Geometry: final body of the model. Coordinates: model frame, mm. Face numbers are marked on the shaded views. Round coordinates to 2 decimals unless told otherwise and drop trailing zeros. Loops run counter-clockwise (first coordinate to the right, second up) from the corner with the lowest first, then second, coordinate; pieces in that order, holes last. Notation, with made-up numbers: (29, -7.75) -> (62, -7.75) arc R9 cw to (62, 4.25) -> close; hole circle Ø5 at (-9.75, 3). An arc over 180 degrees is marked (long way). Answer in a Markdown table with one row per item.
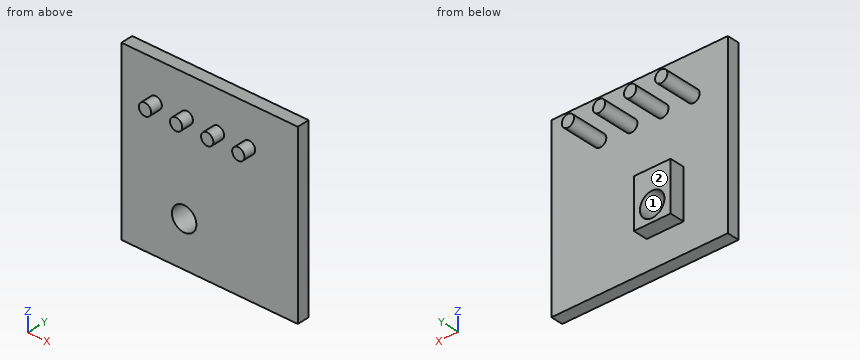
Autodesk Inventor part; units mm, degrees
ref_plane "YZ Plane" through (0, 0, 0) normal (1, 0, 0) x (0, 1, 0)
ref_plane "XZ Plane" through (0, 0, 0) normal (0, 1, 0) x (-1, 0, 0)
ref_plane "XY Plane" through (0, 0, 0) normal (0, 0, 1) x (1, 0, 0)
sketch "Skizze1" plane through (0, 0, 0) normal (0, 1, 0) x (-1, 0, 0)
  line L0 (0, 0) -> (14.4, 0)
  line L1 (14.4, 0) -> (14.4, -14.4)
  line L2 (14.4, -14.4) -> (0, -14.4)
  line L3 (0, -14.4) -> (0, 0)
  dimension "d0" = 14.4
  dimension "d1" = 14.4
extrude "Extrusion1" add sketch "Skizze1" along normal blind 1
sketch "Skizze2" plane through (0, 1, 0) normal (0, 1, 0) x (1, 0, 0)
  line L0 (0, 14.4) -> (-14.4, 14.4)
  line L1 (0, 0) -> (0, 14.4)
  point P0 (-9.28, 10.68)
  dimension "d4" = 3.72
  dimension "d5" = 9.28
hole "Bohrung1" at (-9.28, 1, -10.68) direction (0, -1, 0) diameter 2 end up to surface
sketch "Skizze3" plane through (0, 1, 0) normal (0, 1, 0) x (1, 0, 0)
  circle A0 centre (-9.28, 10.68) radius 1
  line L0 (-14.4, 0) -> (0, 0)
  line L1 (0, 0) -> (0, 14.4)
  line L2 (0, 14.4) -> (-14.4, 14.4)
  line L3 (-14.4, 14.4) -> (-14.4, 0)
  line L4 (-10.78, 8) -> (-7.78, 8)
  line L5 (-7.78, 8) -> (-7.78, 12)
  line L6 (-7.78, 12) -> (-10.78, 12)
  line L7 (-10.78, 12) -> (-10.78, 8)
  dimension "d13" = 4
  dimension "d14" = 3
  dimension "d15" = 1.5
  dimension "d16" = 1.32
extrude "Extrusion2" add sketch "Skizze3" along normal blind 1.2 contours L7 L6 L5 L4
sketch "Skizze4" plane through (0, 1, 0) normal (0, 1, 0) x (1, 0, 0)
  line L0 (-14.4, 14.4) -> (-14.4, 0) construction
  line L1 (-14.4, 3.2) -> (0, 3.2) construction
  line L2 (0, 0) -> (0, 14.4) construction
  line L3 (-14.4, 0) -> (0, 0)
  circle A0 centre (-11.6, 3.2) radius 0.5
  circle A1 centre (-9.06, 3.2) radius 0.5
  circle A2 centre (-6.52, 3.2) radius 0.5
  circle A3 centre (-3.98, 3.2) radius 0.5
  dimension "d19" = 3.2
  dimension "d20" = 2.8
  dimension "d21" = 2.54
  dimension "d22" = 2.54
  dimension "d23" = 2.54
  dimension "d24" = 1
  dimension "d25" = 1
  dimension "d26" = 1
  dimension "d27" = 1
extrude "Extrusion3" add sketch "Skizze4" along normal blind 3 and the other way blind 2
properties part number "Mic_breakout" material "ABS-Kunststoff"
Item 1: Section query D-D, the plane y = 3.4. Output: boundary loops of the cut face in (x, z), and give its area (3 significant figures).
Ans:
| item | result |
|---|---|
| outline | circle Ø1 at (-11.6, -3.2); circle Ø1 at (-9.06, -3.2); circle Ø1 at (-6.52, -3.2); circle Ø1 at (-3.98, -3.2) |
| area | 3.14 mm2 |
Item 2: Ray query, L1, parallel to X at y = 0.9, z = -10.68; L2, parallel to Z at x = -9.28, y = 0.8; L3, parallel to X at y = 3.3, z = -3.5. Return the intervals inside material, ascending.
Ans:
| item | result |
|---|---|
| L1 | -14.4 to -10.28, -8.28 to 0 |
| L2 | -14.4 to -11.68, -9.68 to 0 |
| L3 | -12 to -11.2, -9.46 to -8.66, -6.92 to -6.12, -4.38 to -3.58 |
Item 3: First-contact query: P1, Ø3, axis at x = -10, z = -4.5, coming from the -Y side; P2, Ø1, axis at y = 2, z = -11, coming from the -X side; P3, Ø2.5, axis at x = -9, z = -10, coming from the +Y side; P4, Ø0.6, axis at x = -10, y = 2, coming from the +Z side. Flat tips, straight axial feed; report the tip coordinate or a pass-through.
Ans:
| item | result |
|---|---|
| P1 | y = -1 |
| P2 | x = -10.78 |
| P3 | y = 2.2 |
| P4 | z = -8 |
Item 4: Mould query, pull axis Z, two halves, no side actions, for the marked faces 1 and 2. Classes: released by +Z, released by -Z, zero draft, split by the parting line, or undercut.
Ans:
| item | result |
|---|---|
| face 1 | undercut |
| face 2 | zero draft |
Item 5: Section query A-A, the plane z = -10.68. Output: boundary loops of the cut face in (x, y), and give its area (3 significant figures).
Ans:
| item | result |
|---|---|
| outline | (-14.4, 0) -> (-10.28, 0) -> (-10.28, 2.2) -> (-10.78, 2.2) -> (-10.78, 1) -> (-14.4, 1) -> close; (-8.28, 0) -> (0, 0) -> (0, 1) -> (-7.78, 1) -> (-7.78, 2.2) -> (-8.28, 2.2) -> close |
| area | 13.6 mm2 |
Item 6: Section query C-C, the plane x = -9.06. Output: boundary loops of the cut face in (y, z), and give its area (3 significant figures).
Ans:
| item | result |
|---|---|
| outline | (-1, -3.7) -> (0, -3.7) -> (0, -9.7) -> (2.2, -9.7) -> (2.2, -8) -> (1, -8) -> (1, -3.7) -> (4, -3.7) -> (4, -2.7) -> (1, -2.7) -> (1, 0) -> (0, 0) -> (0, -2.7) -> (-1, -2.7) -> close; (0, -14.4) -> (1, -14.4) -> (1, -12) -> (2.2, -12) -> (2.2, -11.66) -> (0, -11.66) -> close |
| area | 18.9 mm2 |
Item 7: Section query B-B, the plane x = -6.52. Output: boundary loops of the cut face in (y, z), and give its area (3 significant figures).
Ans:
| item | result |
|---|---|
| outline | (-1, -3.7) -> (0, -3.7) -> (0, -14.4) -> (1, -14.4) -> (1, -3.7) -> (4, -3.7) -> (4, -2.7) -> (1, -2.7) -> (1, 0) -> (0, 0) -> (0, -2.7) -> (-1, -2.7) -> close |
| area | 18.4 mm2 |
